```python
from build123d import *

# Parameters (mm, degrees)
SKETCH1_R                = 35
BOSS_EXTRUDE1_DEPTH      = 25
FILLET1_R                = 10
SHELL1_T                 = -3
SKETCH3_R                = 4
BOSS_EXTRUDE2_DEPTH      = 5
CIRPATTERN1_COUNT        = 3
CUT_EXTRUDE1_DEPTH       = 72.991907702
LPATTERN1_COUNT          = 7
LPATTERN1_PITCH          = 6
BOSS_EXTRUDE4_DEPTH      = 5
BOSS_EXTRUDE4_DEPTH_BACK = 5
SKETCH14_R               = 12.5
SKETCH15_R               = 7.5
CUT_EXTRUDE2_DEPTH       = 74.877160033
FILLET3_R                = 2


with BuildPart() as part:
    # Sketch1 → Boss-Extrude1 (new body)
    with BuildSketch(Plane(origin=(0, 0, 0), x_dir=(1, 0, 0), z_dir=(0, 1, 0))):
        with Locations(Location((0, 0, 0), (0, 0, 270))):
            Circle(SKETCH1_R)
    extrude(amount=BOSS_EXTRUDE1_DEPTH)

    # Fillet1
    fillet1_edges = [part.edges().sort_by_distance(p)[0] for p in [
        (0, 25, -35),
    ]]
    fillet(fillet1_edges, radius=FILLET1_R)

    # Shell1
    shell1_openings = [part.faces().sort_by_distance(p)[0] for p in [
        (0, 0, 0),
    ]]
    offset(amount=SHELL1_T, openings=shell1_openings, kind=Kind.INTERSECTION)

    # Sketch3 → Boss-Extrude2 (add)
    with BuildSketch(Plane(origin=(0, 0, 0), x_dir=(1, 0, 0), z_dir=(0, 1, 0))):
        with BuildLine():
            Line((-8, 34.073450075), (8, 34.073450075))
            Line((8, 34.073450075), (8, 42.5))
            ThreePointArc((8, 42.5), (0, 50.5), (-8, 42.5))
            Line((-8, 42.5), (-8, 34.073450075))
        make_face()
        with Locations(Location((0, 42.5, 0), (0, 0, 270))):
            Circle(SKETCH3_R, mode=Mode.SUBTRACT)
    boss_extrude2 = extrude(amount=BOSS_EXTRUDE2_DEPTH)

    # CirPattern1: Boss-Extrude2 ×3 about axis
    cirpattern1_axis = Axis((0, 0, 0), (0, 1, 0))
    for i in range(1, CIRPATTERN1_COUNT):
        add(boss_extrude2.rotate(cirpattern1_axis, i * 360 / CIRPATTERN1_COUNT))

    # Sketch4 → Cut-Extrude1 (cut, through all)
    with BuildSketch(Plane(origin=(0, 25, 0), x_dir=(1, 0, 0), z_dir=(0, 1, 0))):
        with BuildLine():
            Line((-16, 20), (-16, -20))
            ThreePointArc((-16, -20), (-18, -22), (-20, -20))
            Line((-20, -20), (-20, 20))
            ThreePointArc((-20, 20), (-18, 22), (-16, 20))
        make_face()
    cut_extrude1 = extrude(amount=-CUT_EXTRUDE1_DEPTH, mode=Mode.SUBTRACT)

    # LPattern1: Cut-Extrude1 ×7
    with Locations(*[(i * LPATTERN1_PITCH, 0, 0) for i in range(1, LPATTERN1_COUNT)]):
        add(cut_extrude1, mode=Mode.SUBTRACT)

    # Sketch14 → Boss-Extrude4 (add, two sides: drawn at the far end of the back side and taken through both)
    with BuildSketch(Plane(origin=(0, 25, 0), x_dir=(1, 0, 0), z_dir=(0, 1, 0)).offset(-BOSS_EXTRUDE4_DEPTH_BACK)):
        with Locations(Location((0, 0, 0), (0, 0, 270))):
            Circle(SKETCH14_R)
    extrude(amount=BOSS_EXTRUDE4_DEPTH + BOSS_EXTRUDE4_DEPTH_BACK)

    # Sketch15 → Cut-Extrude2 (cut, through all)
    with BuildSketch(Plane(origin=(0, 30, 0), x_dir=(1, 0, 0), z_dir=(0, 1, 0))):
        with Locations(Location((0, 0, 0), (0, 0, 270))):
            Circle(SKETCH15_R)
    extrude(amount=-CUT_EXTRUDE2_DEPTH, mode=Mode.SUBTRACT)

    # Fillet3
    fillet3_edges = [part.edges().sort_by_distance(p)[0] for p in [
        (0, 30, -12.5),
    ]]
    fillet(fillet3_edges, radius=FILLET3_R)


solid = part.part
```
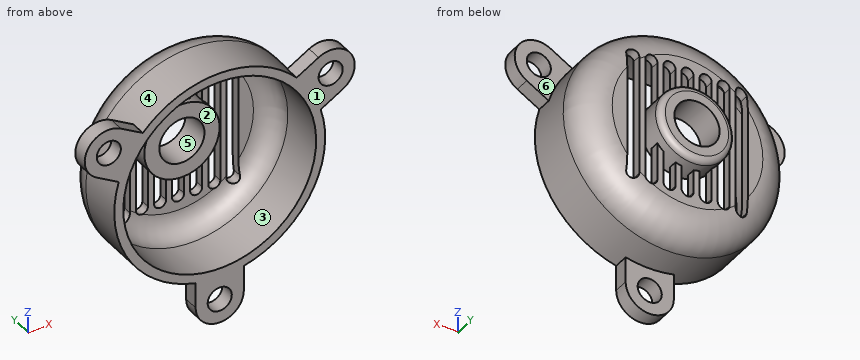
Work out the finished part from the listing and answer in its coordinate system (mm). Face numbers are marked on the shaded views. A direction names the side the tool comes from. Give positions to 0.01 mm unless a question says otherwise; leave off trailing zeros. Loops run counter-clockwise (first coordinate to the right, second up) from the corner with the lowest first, then second, coordinate; pieces in that order, holes last. Notation, with made-up numbers: M 34.25,57.25 L 67.25,57.25 A28 cw 67.25,88.25 Z; hole C 28.25,42 d3. An arc over 180 degrees is marked long. One line per item, written item: value. Start each with the question number.
1. Which of the six approach directions +Z, -Z, +X, -X, +Y, -Y give full straight-line access (tool end or side, diameter ignored) to the marked faces 3, 4, 5 and 6?
2. Find section A-A (x = 0). State how many separate pieces and enclosed holes the cut face has, and give its area (3 significant figures).
3. Each of these flat-tipped pins is pushed along its axis until it touches: P1, Ø5, axis at y = 7, z = 5, coming from the +X side; P2, Ø4, axis at x = 19.5, y = 6.5, coming from the -Z side; P3, Ø3.5, axis at y = 23, z = 15, coming from the -X side. Where does it stop, or does it pass through?
4. Determine the mould class of the marked faces 1 and 2 for opening direction Z: released by +Z, released by -Z, zero draft, split by the parting line, or undercut.
5. Find section D-D (y = 16.5). Give the vertices of the cut face in (x, z).
6. Find section B-B (x = -38). Give the vertices of the cut face in (y, z).
7. Find the intervals of material crossed by probe 1 along X at (y, z) = (2.6, -42.5); probe 2 along X at (y, z) = (26, 0); probe 3 along Z at (x, y) = (5, 20.5), in increasing order.
8. Find section C-C (y = 3.5). Give the vertices of the cut face in (x, z), and give its area (3 significant figures).
Reported:
1. face 3: -Y
1. face 4: +Y
1. face 5: +Y, -Y
1. face 6: +Z, +X, +Y
2. separate pieces: 5
2. enclosed holes: 0
2. area: 324 mm²
3. P1: stops at x = 34.91
3. P2: stops at z = -30.31
3. P3: stops at x = -29.4
4. face 1: zero draft
4. face 2: undercut
5. outline: C 0,0 d69.77; hole C 0,0 d63.67
6. outline: M 0,12.7 L 5,12.7 L 5,17.43 L 0,17.43 Z; M 0,25.07 L 5,25.07 L 5,29.16 L 0,29.16 Z
7. probe 1: x = -8 to -4, 4 to 8
7. probe 2: x = -12.5 to -7.5, 7.5 to 12.5
7. probe 3: z = -32.97 to -28.9, -11.46 to -5.59, 5.59 to 11.46, 28.9 to 32.97
8. outline: M -40.81,14.32 L -33.51,10.11 A35 ccw -8,-34.07 L -8,-42.5 A8 ccw 8,-42.5 L 8,-34.07 A35 ccw 33.51,10.11 L 40.81,14.32 A8 ccw 32.81,28.18 L 25.51,23.96 A35 ccw -25.51,23.96 L -32.81,28.18 A8 ccw Z; hole C -36.81,21.25 d8; hole C 0,0 d64; hole C 0,-42.5 d8; hole C 36.81,21.25 d8
8. area: 1,160 mm²
